The figure shows three views and two pictorial views of one solid part (mm, origin at its lowest corner). Answer the questions. A direction names the side the tool comes from. Coordinates: 2 decimals unless noted, no trailing zeros. Loops run counter-clockwise (first coordinate to the right, second up) from the corner with the lowest first, then second, coordinate; pieces in that order, holes last. Notation, with made-up numbers: M -25.75,40 L 31.25,40 A15 cw 31.25,69 Z; hole C 35.5,24 d7. An arc over 180 degrees is marked long. Return JSON: item names as keys, results as strings. Group by question number.
1. Given P1, Ø11.5, axis at x = 12.7, y = 102.39, coming from the -Z side; P2, Ø10.5, axis at x = 15.5, y = 101, coming from the -Z side; P3, Ø6.5, axis at y = 94, z = 15.5, coming from the +X side; P4, Ø7.5, axis at x = 8, z = 13.5, coming from the +Y side, each flat-ended and moving along its own axis, determine where each tip first touches the part or whether it passes through.
2. Section A-A (x = 18) is taken. Write down the section's boundary in (y, z).
3. Straight lines are drawn through the part: L1, parallel to Y at x = 12.5, z = 18; L2, parallel to Y at x = 11.25, z = 11 (1 decimal); L3, parallel to Z at x = 4.5, y = 102.5. For each, find the intervals that lie inside material, in ascending order. Write a range as from..to.
4. Which of the six approach directions +Z, -Z, +X, -X, +Y, -Y give full straight-line access (tool end or side, diameter ignored) to the marked faces 5, 6 and 7?
5. The mould has two halves that part along X. Classify the marked faces 1, 2, 3 and 4: pulls with the +X half, pulls with the -X half, needs draft (parallel to the pull), parting line crosses it, or undercut.
6. Section D-D (y = 74) is taken. Write down the section's boundary in (x, z).
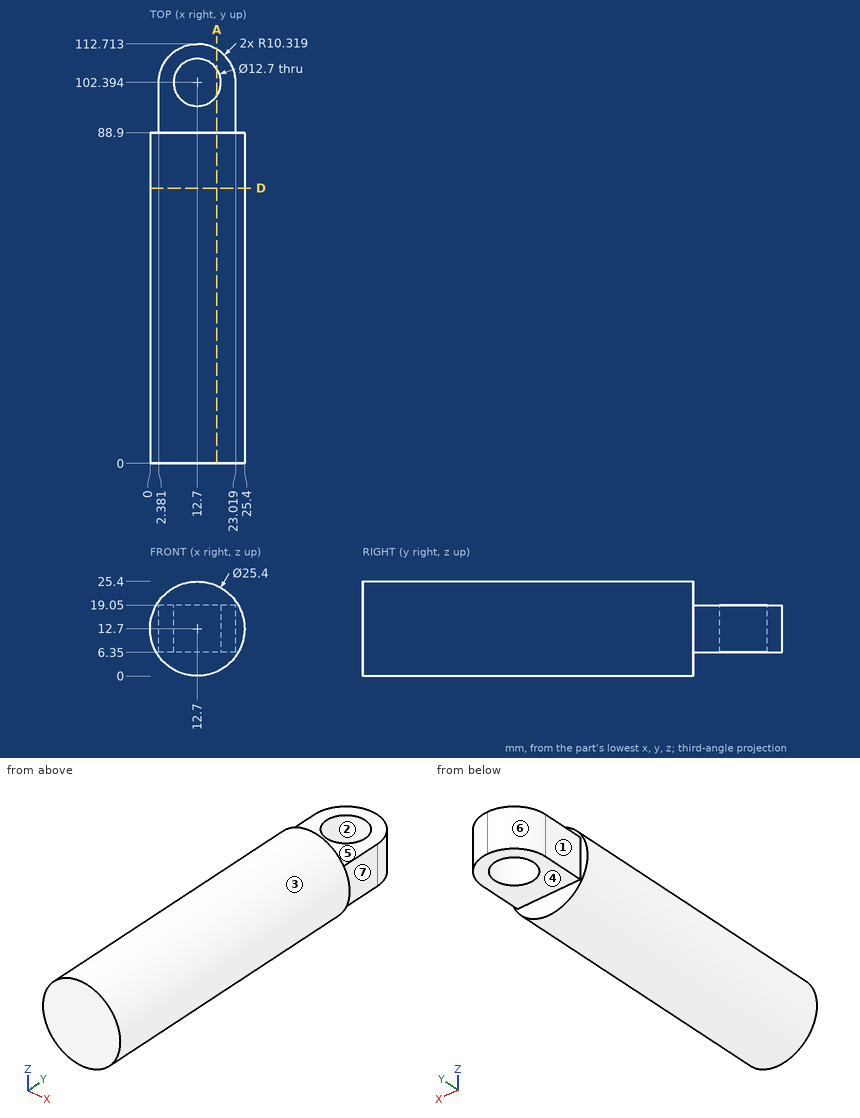
Worked out:
{
 "1": {"P1": "through", "P2": "z = 6.35", "P3": "x = 23.02", "P4": "y = 112.67"},
 "2": {"outline": "M 0,1.16 L 88.9,1.16 L 88.9,6.35 L 98.9,6.35 L 98.9,19.05 L 88.9,19.05 L 88.9,24.24 L 0,24.24 Z; M 105.89,6.35 L 111.25,6.35 L 111.25,19.05 L 105.89,19.05 Z"},
 "3": {"L1": "0..96.05, 108.74..112.71", "L2": "0..96.2, 108.6..112.6", "L3": "6.35..19.05"},
 "4": {"face 5": "+Z, +X, -X, +Y", "face 6": "+Z, -Z, -X, +Y", "face 7": "+Z, -Z, +X, +Y"},
 "5": {"face 1": "pulls with the -X half", "face 2": "undercut", "face 3": "parting line crosses it", "face 4": "needs draft"},
 "6": {"outline": "C 12.7,12.7 d25.4"}
}
